For this review, take the finished solid that the model builds, in its own axes (mm). A direction names the side the tool comes from. Round coordinates to 2 decimals unless told otherwise and drop trailing zeros. Loops run counter-clockwise (first coordinate to the right, second up) from the corner with the lowest first, then second, coordinate; pieces in that order, holes last. Notation, with made-up numbers: (-25.5, -33) -> (-19.5, -33) arc R15 cw to (-19.5, -11) -> close; hole circle Ø6 at (87.25, 84.5). An arc over 180 degrees is marked (long way). Write each question's results on one line, items separated by ' | '.
```python
from build123d import *

# Parameters (mm, degrees)
SKETCH1_W               = 70
SKETCH1_H               = 6
BOSS_EXTRUDE1_DEPTH     = 5
SKETCH5_W               = 4.113429611
SKETCH5_H               = 5.054148352
BOSS_EXTRUDE4_DEPTH     = 40
SKETCH9_W               = 5.188919622
SKETCH9_H               = 2.498562964
CUT_EXTRUDE6_DEPTH      = 6
FILLET14_R              = 1
FILLET15_R              = 1
SKETCH11_R              = 0.939549209
CUT_EXTRUDE8_DEPTH      = 6
FILLET19_R              = 2
SKETCH12_W              = 2.865541581
SKETCH12_H              = 2.859268941
BOSS_EXTRUDE5_DEPTH     = 6
CUT_EXTRUDE9_DEPTH      = 12
CUT_EXTRUDE9_DEPTH_BACK = 5
SKETCH13_W              = 1.424860979
SKETCH13_H              = 2.636738839
SKETCH14_R              = 0.7
CUT_EXTRUDE10_DEPTH     = 13
FILLET20_R              = 1.5


with BuildPart() as part:
    # Sketch1 → Boss-Extrude1 (new body)
    with BuildSketch(Plane.XY):
        Rectangle(SKETCH1_W, SKETCH1_H)
    extrude(amount=BOSS_EXTRUDE1_DEPTH)

    # Sketch5 → Boss-Extrude4 (add)
    with BuildSketch(Plane(origin=(0, 0, 0), x_dir=(0, 0, -1), z_dir=(1, 0, 0))):
        with Locations((-2.56083925, -0.011702819)):
            Rectangle(SKETCH5_W, SKETCH5_H)
    extrude(amount=BOSS_EXTRUDE4_DEPTH)

    # Sketch9 → Cut-Extrude6 (cut)
    with BuildSketch(Plane.XZ.offset(2.538776995)):
        with Locations((37.929941449, 2.575384926)):
            Rectangle(SKETCH9_W, SKETCH9_H)
    extrude(amount=-CUT_EXTRUDE6_DEPTH, mode=Mode.SUBTRACT)

    # Fillet14
    fillet14_edges = [part.edges().sort_by_distance(p)[0] for p in [
        (0, 3, 5),
    ]]
    fillet(fillet14_edges, radius=FILLET14_R)

    # Fillet15
    fillet15_edges = [part.edges().sort_by_distance(p)[0] for p in [
        (0, -3, 5),
        (0, -3, 0),
        (0, 3, 0),
    ]]
    fillet(fillet15_edges, radius=FILLET15_R)

    # Sketch11 → Cut-Extrude8 (cut)
    with BuildSketch(Plane(origin=(0, 0, 0.504124444), x_dir=(-1, 0, 0), z_dir=(0, 0, -1))):
        with Locations((-37.826949183, 0.145030674)):
            Circle(SKETCH11_R)
    extrude(amount=-CUT_EXTRUDE8_DEPTH, mode=Mode.SUBTRACT)

    # Fillet19
    fillet19_edges = [part.edges().sort_by_distance(p)[0] for p in [
        (40, 2.515371357, 0.915113944),
        (40, -2.538776995, 4.221110231),
        (40, 2.515371357, 4.221110231),
        (40, -2.538776995, 0.915113944),
    ]]
    fillet(fillet19_edges, radius=FILLET19_R)

    # Sketch12 → Boss-Extrude5 (add)
    with BuildSketch(Plane(origin=(0, 0, 0), x_dir=(1, 0, 0), z_dir=(0, 1, 0))):
        with Locations((-1.172253324, -2.671686226)):
            Rectangle(SKETCH12_W, SKETCH12_H)
    extrude(amount=BOSS_EXTRUDE5_DEPTH)

    # Sketch13 → Cut-Extrude9 (cut, two sides: drawn at the far end of the back side and taken through both)
    with BuildSketch(Plane(origin=(0, 0, 0), x_dir=(0, 0, -1), z_dir=(1, 0, 0)).offset(-CUT_EXTRUDE9_DEPTH_BACK)):
        with Locations((-2.737982633, 4.937385392)):
            Rectangle(SKETCH13_W, SKETCH13_H)
    extrude(amount=CUT_EXTRUDE9_DEPTH + CUT_EXTRUDE9_DEPTH_BACK, mode=Mode.SUBTRACT)

    # Sketch14 → Cut-Extrude10 (cut)
    with BuildSketch(Plane.XY):
        with Locations(Location((-1.141664566, 4.804714943, 0), (0, 0, 180))):
            Circle(SKETCH14_R)
    extrude(amount=CUT_EXTRUDE10_DEPTH, mode=Mode.SUBTRACT)

    # Fillet20
    # the kernel refuses this fillet: 1.5 mm, written as the material it takes off along each edge
    with BuildSketch(Plane(origin=(0.260517466, 6, 7.851320696), x_dir=(0, -1, 0), z_dir=(0, 0, -1)), Plane(origin=(-2.605024115, 6, -0.299586878), x_dir=(0, -1, 0), z_dir=(0, 0, 1))) as fillet20_piece_1:
        with BuildLine():
            CenterArc((FILLET20_R, FILLET20_R), FILLET20_R, 180, 90)
            Line((0, FILLET20_R), (0, 0))
            Line((0, 0), (FILLET20_R, 0))
        make_face()
    extrude(amount=8.150907574, mode=Mode.SUBTRACT)
    with BuildSketch(Plane(origin=(0.260517466, 6, 5.775552143), x_dir=(0, -1, 0), z_dir=(0, 0, -1)), Plane(origin=(-2.605024115, 6, -2.507948245), x_dir=(0, -1, 0), z_dir=(0, 0, 1))) as fillet20_piece_2:
        with BuildLine():
            CenterArc((FILLET20_R, FILLET20_R), FILLET20_R, 180, 90)
            Line((0, FILLET20_R), (0, 0))
            Line((0, 0), (FILLET20_R, 0))
        make_face()
    extrude(amount=8.283500388, mode=Mode.SUBTRACT)


solid = part.part
```
1. To check wall thickness, follow probe 1 along Y at (x, z) = (-7.5, 2.4); probe 2 along X at (y, z) = (-1.5, 2.9); probe 3 along X at (y, z) = (4, 4.05). State the ranges of each line that lie inside material, in increasing order.
Values found:
probe 1: y = -3 to 3 | probe 2: x = -35 to 35.34 | probe 3: x = -2.61 to 0.26
2. Draft analysis for pull direction Y (two halves, no side actions). For faces 5 (the face through (39.399, -1.968, 0.909)), 6 (the face through (37, -1, 0.504)), 7 (the face through (-0.99, 5.49, 3.77)), 8 (the face through (38.766, 0.186, 4.216)), state which applies: released by +Y, released by -Y, zero draft, split by the parting line, or undercut.
Values found:
face 5: released by -Y | face 6: zero draft | face 7: undercut | face 8: undercut
3. Consider section A-A (x = 11.5). State the section outline as (y, z) points, plus the area to 3 significant figures.
Values found:
outline: (-3, 1) arc R1 ccw to (-2, 0) -> (2, 0) arc R1 ccw to (3, 1) -> (3, 4) arc R1 ccw to (2, 5) -> (-2, 5) arc R1 ccw to (-3, 4) -> close | area: 29.1 mm2
4. Tool access review of faces 1 (the face through (37, -1, 4.618)), 2 (the face through (-2, 4, 4.101)), 3 (the face through (0.261, 3.4, 2.7)), 4 (the face through (-1, 3.619, 3)): name each direction out of +Z, -Z, +X, -X, +Y, -Y from which nothing blocks a thin tool from reaching the whole face with its end or side.
Values found:
face 1: +Z, +X, +Y, -Y | face 2: +Z, +X, -X, +Y | face 3: +Z, -Z, +X, +Y | face 4: +X, -X, +Y
5. For pin 1 (3 mm diameter, centred on x = -21, z = 1.5, fed in from +Y); pin 2 (2.5 mm diameter, centred on x = -1, y = 4.5, fed in from -Z); pin 3 (2.5 mm diameter, centred on x = 36.5, z = 2.5, fed in from +Y), all flat-tipped, find the tip position at first contact; note any pin that passes through.
Values found:
pin 1: stops at y = 3 | pin 2: stops at z = 1.24 | pin 3: stops at y = 2.52
